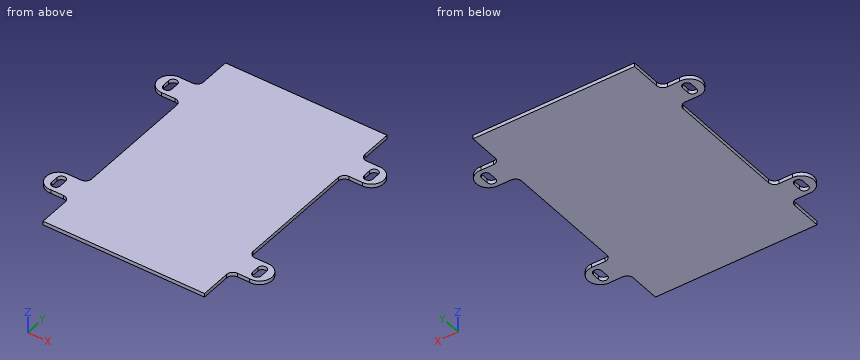
from build123d import *

# Parameters (mm, degrees)
BOSS_EXTRUDE1_DEPTH = 3


with BuildPart() as part:
    # Sketch2 → Boss-Extrude1 (new body)
    with BuildSketch(Plane.XY):
        with BuildLine():
            Line((-65.5, -103), (65.5, -103))
            Line((65.5, -103), (65.5, -78))
            ThreePointArc((65.5, -78), (66.964466094, -74.464466094), (70.5, -73))
            Line((70.5, -73), (80.5, -73))
            ThreePointArc((80.5, -73), (91.487460731, -63.55075338), (81.5, -53.050125629))
            Line((81.5, -53.050125629), (70.5, -53.050125629))
            ThreePointArc((70.5, -53.050125629), (66.964466094, -51.585659535), (65.5, -48.050125629))
            Line((65.5, -48.050125629), (65.5, 48.050125629))
            ThreePointArc((65.5, 48.050125629), (66.964466094, 51.585659535), (70.5, 53.050125629))
            Line((70.5, 53.050125629), (81.5, 53.050125629))
            ThreePointArc((81.5, 53.050125629), (91.487460731, 63.55075338), (80.5, 73))
            Line((80.5, 73), (70.5, 73))
            ThreePointArc((70.5, 73), (66.964466094, 74.464466094), (65.5, 78))
            Line((65.5, 78), (65.5, 103))
            Line((65.5, 103), (-65.5, 103))
            Line((-65.5, 103), (-65.5, 78))
            ThreePointArc((-65.5, 78), (-66.964466094, 74.464466094), (-70.5, 73))
            Line((-70.5, 73), (-80.5, 73))
            ThreePointArc((-80.5, 73), (-91.487460731, 63.55075338), (-81.5, 53.050125629))
            Line((-81.5, 53.050125629), (-70.5, 53.050125629))
            ThreePointArc((-70.5, 53.050125629), (-66.964466094, 51.585659535), (-65.5, 48.050125629))
            Line((-65.5, 48.050125629), (-65.5, -48.050125629))
            ThreePointArc((-65.5, -48.050125629), (-66.964466094, -51.585659535), (-70.5, -53.050125629))
            Line((-70.5, -53.050125629), (-81.5, -53.050125629))
            ThreePointArc((-81.5, -53.050125629), (-91.487460731, -63.55075338), (-80.5, -73))
            Line((-80.5, -73), (-70.5, -73))
            ThreePointArc((-70.5, -73), (-66.964466094, -74.464466094), (-65.5, -78))
            Line((-65.5, -78), (-65.5, -103))
        make_face()
        with BuildLine():
            Line((78, 60.050125629), (78, 66.050125629))
            ThreePointArc((78, 66.050125629), (81.5, 69.550125629), (85, 66.050125629))
            Line((85, 66.050125629), (85, 60.050125629))
            ThreePointArc((85, 60.050125629), (81.5, 56.550125629), (78, 60.050125629))
        make_face(mode=Mode.SUBTRACT)
        with BuildLine():
            Line((-78, 60.050125629), (-78, 66.050125629))
            ThreePointArc((-78, 66.050125629), (-81.5, 69.550125629), (-85, 66.050125629))
            Line((-85, 66.050125629), (-85, 60.050125629))
            ThreePointArc((-85, 60.050125629), (-81.5, 56.550125629), (-78, 60.050125629))
        make_face(mode=Mode.SUBTRACT)
        with BuildLine():
            Line((-78, -60.050125629), (-78, -66.050125629))
            ThreePointArc((-78, -66.050125629), (-81.5, -69.550125629), (-85, -66.050125629))
            Line((-85, -66.050125629), (-85, -60.050125629))
            ThreePointArc((-85, -60.050125629), (-81.5, -56.550125629), (-78, -60.050125629))
        make_face(mode=Mode.SUBTRACT)
        with BuildLine():
            Line((78, -60.050125629), (78, -66.050125629))
            ThreePointArc((78, -66.050125629), (81.5, -69.550125629), (85, -66.050125629))
            Line((85, -66.050125629), (85, -60.050125629))
            ThreePointArc((85, -60.050125629), (81.5, -56.550125629), (78, -60.050125629))
        make_face(mode=Mode.SUBTRACT)
    extrude(amount=BOSS_EXTRUDE1_DEPTH)


solid = part.part
Work out the finished part from the listing and answer in its coordinate system (mm). Round coordinates to 2 decimals unless told otherwise and drop trailing zeros. Order: outer loops, then holes, each group sorted by start corner. A loop starts at its lowest first (then second) coordinate and runs counter-clockwise, first axis right, second up. Notation, with made-up numbers: M 10,48.5 L 54,48.5 A21 ccw 54,79.5 Z; hole C 0,32.5 d4. An arc over 180 degrees is marked long. Put each result on its own line as item: value. Start each with the question number.
Q1. Section B-B, the plane y = 2.5 is taken. Write down the section's boundary in (x, z), and give its area (3 significant figures).
Q2. Straight lines are drawn through the part: L1, parallel to X at y = 63.5, z = 2.15; L2, parallel to Y at x = -77, z = 1.5; L3, parallel to X at y = 31, z = 0.55. For each, find the intervals that lie inside material, in ascending order. Write a range as [from, to].
Q3. Section A-A, the plane z = 1.7 is taken. Give the number of separate pieces and of enclosed holes in the cut face, and give its area (3 significant figures).
Q4. Flat-ended cylindrical pins translate along their axes: pin 1 (1.5 mm diameter, centred on x = 73.5, z = 1.5, fed in from -Y); pin 2 (0.9 mm diameter, centred on x = 77.5, z = 1.5, fed in from +Y); pin 3 (0.9 mm diameter, centred on y = -64.5, z = 1.5, fed in from -X). Find the tip coordinate at first contact, or state that the pin passes through.
Findings below:
1. outline: M -65.5,0 L 65.5,0 L 65.5,3 L -65.5,3 Z
1. area: 393 mm^2
2. L1: x = [-91.49, -85], [-78, 78], [85, 91.49]
2. L2: y = [-73, -53.05], [53.05, 73]
2. L3: x = [-65.5, 65.5]
3. separate pieces: 1
3. enclosed holes: 4
3. area: 28,600 mm^2
4. pin 1: stops at y = -73
4. pin 2: stops at y = 73
4. pin 3: stops at x = -91.45
